Part model, mm, in its own coordinate system. A direction names the side the tool comes from. Give positions to 0.01 mm unless a question says otherwise; leave off trailing zeros. Write each loop counter-clockwise with the first axis right and the second up, starting at its lowest first coordinate (ties: lowest second). Pieces come first, ordered by that corner, then holes.
Autodesk Inventor part; units mm, degrees
ref_plane "YZ Plane" through (0, 0, 0) normal (1, 0, 0) x (0, 1, 0)
ref_plane "XZ Plane" through (0, 0, 0) normal (0, 1, 0) x (-1, 0, 0)
ref_plane "XY Plane" through (0, 0, 0) normal (0, 0, 1) x (1, 0, 0)
sketch "Sketch1" plane through (0, 0, 0) normal (0, 0, 1) x (1, 0, 0)
  line L0 (0, 0) -> (30, 0)
  line L1 (30, 0) -> (30, 10.5)
  line L2 (30, 10.5) -> (0, 10.5)
  line L3 (0, 10.5) -> (0, 0)
  circle A0 centre (15.5, 5.25) radius 1.6
  point P0 (0, 5.25)
  dimension "d0" = 30
  dimension "d1" = 10.5
  dimension "d2" = 3.2
  dimension "d3" = 14.5
extrude "Extrusion1" add sketch "Sketch1" along normal blind 1.5
sketch "Sketch2" plane through (0, 0, 1.5) normal (0, 0, 1) x (1, 0, 0)
  line L0 (0, 0) -> (0, 10.5)
  line L1 (30, 10.5) -> (30, 0)
  line L2 (-6, 9.4) -> (2.5, 9.4)
  line L3 (2.5, 9.4) -> (2.5, 1.1)
  line L4 (2.5, 1.1) -> (-6, 1.1)
  line L5 (-6, 1.1) -> (-6, 9.4)
  point P0 (-6, 5.25)
  point P1 (0, 5.25)
  dimension "d6" = 36
  dimension "d7" = 8.3
  dimension "d8" = 2.5
extrude "Extrusion2" add sketch "Sketch2" along normal blind 5
sketch "Sketch3" plane through (0, 0, 0) normal (0, 0, -1) x (-1, 0, 0)
  line L0 (-30, 0) -> (-30, 10.5)
  line L1 (-29.5, 8) -> (-19.5, 8)
  line L2 (-19.5, 8) -> (-19.5, 2.5)
  line L3 (-19.5, 2.5) -> (-29.5, 2.5)
  line L4 (-29.5, 2.5) -> (-29.5, 8)
  point P0 (-29.5, 5.25)
  point P1 (-30, 5.25)
  dimension "d11" = 10
  dimension "d12" = 5.5
  dimension "d13" = 0.5
extrude "Extrusion3" add sketch "Sketch3" along normal blind 8
properties part number "Sensor"
1) Flat gauge pins, fed straight in: P1, Ø1.5, axis at x = -4, z = 3.5, coming from the -Y side; P2, Ø2.5, axis at y = 4.5, z = 4, coming from the +X side; P3, Ø3.5, axis at x = 15.5, y = 5.25, coming from the -Z side; P4, Ø1.2, axis at y = 7, z = 1, coming from the -X side. Where does each tip first touch, or does it go through?
Check result:
P1: stops at y = 1.1
P2: stops at x = 2.5
P3: stops at z = 0
P4: stops at x = -6
2) Mould opens along X. For faces 6 (the flat face through (18, 5, 1.5)), 7 (the cylindrical face through (13.9, 5.2, 0.7)), 8 (the flat face through (19.5, 5, -4)) say: +X half, -X half, draft (parallel to the pull), parting line (faces both ways), or undercut.
Check result:
face 6: draft
face 7: undercut
face 8: -X half
3) Drill centre lines: L1, parallel to Y at x = 15.5, z = 0.8; L2, parallel to Z at x = 5, y = 6.75; L3, parallel to Z at x = -2.5, y = 3.5. Where is each one in solid material? Low to high.
Check result:
L1: y = 0 to 3.65, 6.85 to 10.5
L2: z = 0 to 1.5
L3: z = 1.5 to 6.5
4) Saw through at C-C (x = 20). Write the cut outline in (y, z).
Check result:
outline: (0, 0) - (2.5, 0) - (2.5, -8) - (8, -8) - (8, 0) - (10.5, 0) - (10.5, 1.5) - (0, 1.5) - close
5) Saw through at D-D (y = 8.75). Write the cut outline in (x, z), and give its area (3 significant figures).
Check result:
outline: (-6, 1.5) - (0, 1.5) - (0, 0) - (30, 0) - (30, 1.5) - (2.5, 1.5) - (2.5, 6.5) - (-6, 6.5) - close
area: 87.5 mm2
6) 3-axis set-ups, long thin cutter, end or side, ignore diameter. For faces 1 (the flat face through (-2, 1.1, 4)), 2 (the flat face through (2.5, 5, 4)), 3 (the flat face through (0, 5, 1)), 4 (the flat face through (29.5, 5, -4)), 5 (the flat face through (24, 2.5, -4)): which of +Z, -Z, +X, -X, +Y, -Y reach the whole face in a straight line?
Check result:
face 1: +Z, +X, -X, -Y
face 2: +Z, +X, +Y, -Y
face 3: -Z, -X, +Y, -Y
face 4: -Z, +X, +Y, -Y
face 5: -Z, +X, -X, -Y
7) Saw through at A-A (x = 15.5). Write the cut outline in (y, z).
Check result:
outline: (0, 0) - (3.65, 0) - (3.65, 1.5) - (0, 1.5) - close; (6.85, 0) - (10.5, 0) - (10.5, 1.5) - (6.85, 1.5) - close
8) Saw through at B-B (y = 5.25). Write the cut outline in (x, z).
Check result:
outline: (-6, 1.5) - (0, 1.5) - (0, 0) - (13.9, 0) - (13.9, 1.5) - (2.5, 1.5) - (2.5, 6.5) - (-6, 6.5) - close; (17.1, 0) - (19.5, 0) - (19.5, -8) - (29.5, -8) - (29.5, 0) - (30, 0) - (30, 1.5) - (17.1, 1.5) - close
